Geometry check sheet. Reference: the model listing, model coordinates, mm. A direction names the side the tool comes from. Coordinates: 2 decimals unless noted, no trailing zeros. Write each loop counter-clockwise with the first axis right and the second up, starting at its lowest first coordinate (ties: lowest second). Pieces come first, ordered by that corner, then holes. Notation, with made-up numbers: (12, -38.5) - (46, -38.5) arc R30 cw to (46, -0.5) - close; hole circle Ø5 at (-20, -24). An arc over 180 degrees is marked (long way). Answer as a JSON object with one key per item and string values. Group by question number.
from build123d import *

# Parameters (mm, degrees)
F1_DEPTH      = 150
F2_W          = 57.983538
F2_H          = 25.869577
F3_DEPTH      = 26
F3_DEPTH_BACK = 32
F4_R          = 19.313708
F5_R          = 5


with BuildPart() as f1:
    # F0 (on Front) → F1 (new body)
    with BuildSketch(Plane.XZ):
        Polygon((-16.769175, 1.928175), (0.331647, -22.070456), (17.145061, 2.359288), (-0.707533, 17.782993), align=None)
    extrude(amount=F1_DEPTH)

    # F2 (on Top) → F3 (join, two sides)
    with BuildSketch(Plane.XY) as f3_sk:
        with Locations((0.403912, -1.548561)):
            Rectangle(F2_W, F2_H)
    extrude(amount=F3_DEPTH)
    extrude(f3_sk.sketch, amount=-F3_DEPTH_BACK)

    # F4
    f4_edges = [f1.edges().sort_by_distance(p)[0] for p in [
        (-28.587857, -1.548562, -32),
        (29.395681, -1.548562, -32),
        (29.395681, -1.548562, 26),
        (-28.587857, -1.548562, 26),
    ]]
    fillet(f4_edges, radius=F4_R)

    # F5
    f5_edges = [f1.edges().sort_by_distance(p)[0] for p in [
        (8.218764, -150, 10.071141),
        (8.738354, -150, -9.855584),
        (-8.738354, -150, 9.855584),
        (-8.218764, -150, -10.071141),
    ]]
    fillet(f5_edges, radius=F5_R)


solid = f1.part
(1) Material ranges on L1, parallel to Z at x = -9.5, y = -11.5; L2, parallel to Y at x = -12, z = -5.5; L3, parallel to X at y = -39, z = 14.5, recorded low to high. Write a range as [from, to].
(2) Section check A-A (y = -1.5). Record the cut outline in (x, z), and give its area (3 significant figures).
(3) Set-up check for faces 1 (the face through (-8.626, -78.828, 9.967)), 2 (the face through (-8.34, -78.83, -9.9)), 3 (the face through (8.3, -78.8, 10)), 4 (the face through (8.62, -78.83, -10.03)), 5 (the face through (6, -14.483, -15)): record each of +Z, -Z, +X, -X, +Y, -Y from which the full face is reachable in a straight line by a thin tool's end or side.
(4) Section check C-C (x = 22). Record the cut outline in (y, z), and give its area (3 significant figures).
(5) Section check B-B (z = -26). Record the cut outline in (x, y).
(6) Gauge pin test, flat ends, axial feed: pin 1 (12 mm diameter, centred on x = -17, y = -91, fed in from +Z); pin 2 (1 mm diameter, centred on x = -17, y = -67.5, fed in from +Z); pin 3 (1.5 mm diameter, centred on x = -5.5, y = -99.5, fed in from +Z). Record the tip position at first contact, or that the pin passes through.
Conclusion:
{
 "1": {"L1": "z = [-32, 26]", "L2": "y = [-14.48, 11.39]", "L3": "x = [-4.03, 3.09]"},
 "2": {"outline": "(-28.59, -12.69) arc R19.31 ccw to (-9.27, -32) - (10.08, -32) arc R19.31 ccw to (29.4, -12.69) - (29.4, 6.69) arc R19.31 ccw to (10.08, 26) - (-9.27, 26) arc R19.31 ccw to (-28.59, 6.69) - close", "area": "3,040 mm^2"},
 "3": {"face 1": "+Z, -X, -Y", "face 2": "-Z, -X, -Y", "face 3": "+Z, +X, -Y", "face 4": "-Z, +X, -Y", "face 5": "-Y"},
 "4": {"outline": "(-14.48, -27.88) - (11.39, -27.88) - (11.39, 21.88) - (-14.48, 21.88) - close", "area": "1,290 mm^2"},
 "5": {"outline": "(-23.27, -14.48) - (24.07, -14.48) - (24.07, 11.39) - (-23.27, 11.39) - close"},
 "6": {"pin 1": "stops at z = 7.62", "pin 2": "stops at z = 2.19", "pin 3": "stops at z = 13.79"}
}
